```python
from build123d import *

# Parameters (mm, degrees)
SALIENTE_EXTRUIR1_DEPTH = 5
SALIENTE_EXTRUIR2_DEPTH = 10
SALIENTE_EXTRUIR3_DEPTH = 2
CORTAR_EXTRUIR1_START   = 7
CROQUIS2_R              = 2.2
CORTAR_EXTRUIR1_DEPTH   = 14
CROQUIS3_R              = 1.6
CROQUIS3_W              = 5
CROQUIS3_H              = 4
CROQUIS3_W_2            = 2
CORTAR_EXTRUIR2_DEPTH   = 2.4
REDONDEO1_R             = 2
REDONDEO2_R             = 2
REDONDEO3_R             = 1
REDONDEO4_R             = 1.2


with BuildPart() as part:
    # Croquis1 → Saliente-Extruir1 (new body)
    with BuildSketch(Plane(origin=(0, 0, 0), x_dir=(0, 0, -1), z_dir=(1, 0, 0))):
        Polygon((-12.7, 2.4), (-12.7, 0), (12.7, 0), (12.7, 2.4), (7, 2.4), (7, 20), (2, 20), (2, 11.4), (4.4, 11.4), (4.4, 8.6), (2, 8.6), (2, 2.4), (-2, 2.4), (-2, 8.6), (-4.4, 8.6), (-4.4, 11.4), (-2, 11.4), (-2, 20), (-7, 20), (-7, 2.4), align=None)
    extrude(amount=-SALIENTE_EXTRUIR1_DEPTH)

    # Croquis1<3> → Saliente-Extruir2 (add)
    with BuildSketch(Plane(origin=(0, 0, 0), x_dir=(0, 0, -1), z_dir=(1, 0, 0))):
        Polygon((2, 2.4), (7, 2.4), (12.7, 2.4), (12.7, 0), (-12.7, 0), (-12.7, 2.4), (-7, 2.4), (-2, 2.4), align=None)
    extrude(amount=SALIENTE_EXTRUIR2_DEPTH)

    # Croquis1<4> → Saliente-Extruir3 (add)
    with BuildSketch(Plane(origin=(0, 0, 0), x_dir=(0, 0, -1), z_dir=(1, 0, 0))):
        Polygon((-7, 20), (-7, 2.4), (-2, 2.4), (-2, 8.6), (-4.4, 8.6), (-4.4, 11.4), (-2, 11.4), (-2, 20), align=None)
        Polygon((2, 2.4), (7, 2.4), (7, 20), (2, 20), (2, 11.4), (4.4, 11.4), (4.4, 8.6), (2, 8.6), align=None)
    extrude(amount=SALIENTE_EXTRUIR3_DEPTH)

    # Croquis2 → Cortar-Extruir1 (cut)
    with BuildSketch(Plane.XY.offset(CORTAR_EXTRUIR1_START)):
        with Locations(Location((-2, 15, 0), (0, 0, 270))):
            Circle(CROQUIS2_R)
        with Locations(Location((-2, 5, 0), (0, 0, 270))):
            Circle(CROQUIS2_R)
    extrude(amount=-CORTAR_EXTRUIR1_DEPTH, mode=Mode.SUBTRACT)

    # Croquis3 → Cortar-Extruir2 (cut)
    with BuildSketch(Plane(origin=(0, 0, 0), x_dir=(1, 0, 0), z_dir=(0, 1, 0))):
        Polygon((-5, 7), (0, 7), (2, 12.7), (-5, 12.7), align=None)
        Polygon((2, -12.7), (0, -7), (-5, -7), (-5, -12.7), align=None)
        with Locations(Location((6, -8.7, 0), (0, 0, 90))):
            Circle(CROQUIS3_R)
        with Locations(Location((6, 8.7, 0), (0, 0, 90))):
            Circle(CROQUIS3_R)
        with Locations((-2.5, 0)):
            Rectangle(CROQUIS3_W, CROQUIS3_H)
        with Locations((1, 0)):
            Rectangle(CROQUIS3_W_2, CROQUIS3_H)
    extrude(amount=CORTAR_EXTRUIR2_DEPTH, mode=Mode.SUBTRACT)

    # Redondeo1
    redondeo1_edges = [part.edges().sort_by_distance(p)[0] for p in [
        (2, 20, -4.5),
        (2, 20, 4.5),
    ]]
    fillet(redondeo1_edges, radius=REDONDEO1_R)

    # Redondeo2
    # the kernel refuses this fillet: 2 mm, written as the material it adds along each edge
    with BuildSketch(Plane(origin=(2, 2.4, 3), x_dir=(1, 0, 0), z_dir=(0, 0, -1))) as redondeo2_piece_1_section:
        with BuildLine():
            CenterArc((REDONDEO2_R, -REDONDEO2_R), REDONDEO2_R, 90, 90)
            Line((0, -REDONDEO2_R), (0, 0))
            Line((0, 0), (REDONDEO2_R, 0))
        make_face()
    redondeo2_piece_1 = extrude(amount=15, mode=Mode.PRIVATE)
    redondeo2_piece_1 = split(redondeo2_piece_1, bisect_by=Plane(origin=(2, 2.4, 2), z_dir=(0, 0, 1)), keep=Keep.TOP, mode=Mode.PRIVATE)
    add(redondeo2_piece_1)
    with BuildSketch(Plane(origin=(2, 2.4, -2), x_dir=(1, 0, 0), z_dir=(0, 0, -1))) as redondeo2_piece_2:
        with BuildLine():
            CenterArc((REDONDEO2_R, -REDONDEO2_R), REDONDEO2_R, 90, 90)
            Line((0, -REDONDEO2_R), (0, 0))
            Line((0, 0), (REDONDEO2_R, 0))
        make_face()
    extrude(amount=5)
    with BuildSketch(Plane(origin=(-5, 2.4, -7), x_dir=(0, 0, -1), z_dir=(1, 0, 0))) as redondeo2_piece_3_section:
        with BuildLine():
            CenterArc((REDONDEO2_R, REDONDEO2_R), REDONDEO2_R, 180, 90)
            Line((0, REDONDEO2_R), (0, 0))
            Line((0, 0), (REDONDEO2_R, 0))
        make_face()
    redondeo2_piece_3 = extrude(amount=7, mode=Mode.PRIVATE)
    redondeo2_piece_3 = split(redondeo2_piece_3, bisect_by=Plane(origin=(-0.548095369, 2.4, -5.4379282), z_dir=(0.9435999821328808, 0, 0.331087713029081)), keep=Keep.TOP, mode=Mode.PRIVATE)
    redondeo2_piece_3 = redondeo2_piece_3 - Plane(origin=(-2, 5, -7), x_dir=(0, -1, 0), z_dir=(0, 0, 1)) * Cylinder(2.2, 22, mode=Mode.PRIVATE)
    add(redondeo2_piece_3)
    with BuildSketch(Plane(origin=(2, 2.4, 7), x_dir=(0, 1, 0), z_dir=(-1, 0, 0))) as redondeo2_piece_4_section:
        with BuildLine():
            CenterArc((REDONDEO2_R, -REDONDEO2_R), REDONDEO2_R, 90, 90)
            Line((0, -REDONDEO2_R), (0, 0))
            Line((0, 0), (REDONDEO2_R, 0))
        make_face()
    redondeo2_piece_4 = extrude(amount=7, mode=Mode.PRIVATE)
    redondeo2_piece_4 = split(redondeo2_piece_4, bisect_by=Plane(origin=(0.219238147, 2.4, 7.62482872), z_dir=(0.9435999821328808, 0, -0.331087713029081)), keep=Keep.TOP, mode=Mode.PRIVATE)
    redondeo2_piece_4 = redondeo2_piece_4 - Plane(origin=(-2, 5, 7), x_dir=(0, -1, 0), z_dir=(0, 0, 1)) * Cylinder(2.2, 22, mode=Mode.PRIVATE)
    add(redondeo2_piece_4)
    with BuildSketch(Plane(origin=(0, 0, 7), x_dir=(-1, 0, 0), z_dir=(0, 1, 0))) as redondeo2_piece_5:
        with BuildLine():
            CenterArc((REDONDEO2_R * 0.708893916529, REDONDEO2_R), REDONDEO2_R, 199.334808538, 70.665191462)
            Line((-REDONDEO2_R * 0.234706065604, REDONDEO2_R * 0.668912286971), (0, 0))
            Line((0, 0), (REDONDEO2_R * 0.708893916529, 0))
        make_face()
    extrude(amount=2.4)
    with BuildSketch(Plane(origin=(0, 0, -7), x_dir=(-1, 0, 0), z_dir=(0, 1, 0))) as redondeo2_piece_6:
        with BuildLine():
            CenterArc((REDONDEO2_R * 0.708893916529, -REDONDEO2_R), REDONDEO2_R, 90, 70.665191462)
            Line((-REDONDEO2_R * 0.234706065604, -REDONDEO2_R * 0.668912286971), (0, 0))
            Line((0, 0), (REDONDEO2_R * 0.708893916529, 0))
        make_face()
    extrude(amount=2.4)
    with BuildSketch(Plane(origin=(2, 2.4, 7), x_dir=(0, 1, 0), z_dir=(0, 0, -1))) as redondeo2_piece_7:
        with BuildLine():
            CenterArc((REDONDEO2_R, REDONDEO2_R), REDONDEO2_R, 180, 90)
            Line((0, REDONDEO2_R), (0, 0))
            Line((0, 0), (REDONDEO2_R, 0))
        make_face()
    extrude(amount=5)
    with BuildSketch(Plane(origin=(2, 2.4, 12), x_dir=(0, 1, 0), z_dir=(0, 0, -1))) as redondeo2_piece_8_section:
        with BuildLine():
            CenterArc((REDONDEO2_R, REDONDEO2_R), REDONDEO2_R, 180, 90)
            Line((0, REDONDEO2_R), (0, 0))
            Line((0, 0), (REDONDEO2_R, 0))
        make_face()
    redondeo2_piece_8 = extrude(amount=15, mode=Mode.PRIVATE)
    redondeo2_piece_8 = split(redondeo2_piece_8, bisect_by=Plane(origin=(2, 2.4, -2), z_dir=(0, 0, -1)), keep=Keep.TOP, mode=Mode.PRIVATE)
    add(redondeo2_piece_8)
    with BuildSketch(Plane(origin=(2, 2.4, -2), x_dir=(1, 0, 0), z_dir=(0, 0, -1))) as redondeo2_piece_9a_section:
        with BuildLine():
            CenterArc((REDONDEO2_R, -REDONDEO2_R), REDONDEO2_R, 90, 90)
            Line((0, -REDONDEO2_R), (0, 0))
            Line((0, 0), (REDONDEO2_R, 0))
        make_face()
    redondeo2_piece_9a = extrude(amount=10, mode=Mode.PRIVATE)
    redondeo2_piece_9a = split(redondeo2_piece_9a, bisect_by=Plane(origin=(2, 2.4, -7), z_dir=(0, 0, -1)), keep=Keep.TOP, mode=Mode.PRIVATE)
    with BuildSketch(Plane(origin=(-5, 2.4, -7), x_dir=(0, 0, -1), z_dir=(1, 0, 0))) as redondeo2_piece_9b_section:
        with BuildLine():
            CenterArc((REDONDEO2_R, REDONDEO2_R), REDONDEO2_R, 180, 90)
            Line((0, REDONDEO2_R), (0, 0))
            Line((0, 0), (REDONDEO2_R, 0))
        make_face()
    redondeo2_piece_9b = extrude(amount=12, mode=Mode.PRIVATE)
    redondeo2_piece_9b = split(redondeo2_piece_9b, bisect_by=Plane(origin=(2, 2.4, -7), z_dir=(1, 0, 0)), keep=Keep.TOP, mode=Mode.PRIVATE)
    redondeo2_piece_9b = redondeo2_piece_9b - Plane(origin=(6, 2.4, -8.7), x_dir=(0, 0, -1), z_dir=(0, -1, 0)) * Cylinder(1.6, 32, mode=Mode.PRIVATE)
    redondeo2_piece_9 = redondeo2_piece_9a & redondeo2_piece_9b
    add(redondeo2_piece_9)
    with BuildSketch(Plane(origin=(-5, 2.4, -7), x_dir=(0, 0, -1), z_dir=(1, 0, 0))) as redondeo2_piece_10a_section:
        with BuildLine():
            CenterArc((REDONDEO2_R, REDONDEO2_R), REDONDEO2_R, 180, 90)
            Line((0, REDONDEO2_R), (0, 0))
            Line((0, 0), (REDONDEO2_R, 0))
        make_face()
    redondeo2_piece_10a = extrude(amount=7, mode=Mode.PRIVATE)
    redondeo2_piece_10a = split(redondeo2_piece_10a, bisect_by=Plane(origin=(-0.548095369, 2.4, -5.4379282), z_dir=(-0.9435999821328808, 0, -0.331087713029081)), keep=Keep.TOP, mode=Mode.PRIVATE)
    redondeo2_piece_10a = redondeo2_piece_10a - Plane(origin=(-2, 5, -7), x_dir=(0, -1, 0), z_dir=(0, 0, 1)) * Cylinder(2.2, 22, mode=Mode.PRIVATE)
    with BuildSketch(Plane(origin=(0, 0, -7), x_dir=(-1, 0, 0), z_dir=(0, 1, 0))) as redondeo2_piece_10b_section:
        with BuildLine():
            CenterArc((REDONDEO2_R * 0.708893916529, -REDONDEO2_R), REDONDEO2_R, 90, 70.665191462)
            Line((-REDONDEO2_R * 0.234706065604, -REDONDEO2_R * 0.668912286971), (0, 0))
            Line((0, 0), (REDONDEO2_R * 0.708893916529, 0))
        make_face()
    redondeo2_piece_10b = extrude(amount=5.944469583, mode=Mode.PRIVATE)
    redondeo2_piece_10b = split(redondeo2_piece_10b, bisect_by=Plane(origin=(0, 2.4, -7), z_dir=(0, 1, 0)), keep=Keep.TOP, mode=Mode.PRIVATE)
    redondeo2_piece_10b = redondeo2_piece_10b - Plane(origin=(-2, 5, -7), x_dir=(0, -1, 0), z_dir=(0, 0, 1)) * Cylinder(2.2, 18, mode=Mode.PRIVATE)
    redondeo2_piece_10 = redondeo2_piece_10a & redondeo2_piece_10b
    add(redondeo2_piece_10)
    with BuildSketch(Plane(origin=(7, 2.4, 7), x_dir=(0, 1, 0), z_dir=(-1, 0, 0))) as redondeo2_piece_11a_section:
        with BuildLine():
            CenterArc((REDONDEO2_R, -REDONDEO2_R), REDONDEO2_R, 90, 90)
            Line((0, -REDONDEO2_R), (0, 0))
            Line((0, 0), (REDONDEO2_R, 0))
        make_face()
    redondeo2_piece_11a = extrude(amount=12, mode=Mode.PRIVATE)
    redondeo2_piece_11a = split(redondeo2_piece_11a, bisect_by=Plane(origin=(2, 2.4, 7), z_dir=(1, 0, 0)), keep=Keep.TOP, mode=Mode.PRIVATE)
    redondeo2_piece_11a = redondeo2_piece_11a - Plane(origin=(6, 2.4, 8.7), x_dir=(0, 0, -1), z_dir=(0, -1, 0)) * Cylinder(1.6, 32, mode=Mode.PRIVATE)
    with BuildSketch(Plane(origin=(2, 2.4, 12), x_dir=(0, 1, 0), z_dir=(0, 0, -1))) as redondeo2_piece_11b_section:
        with BuildLine():
            CenterArc((REDONDEO2_R, REDONDEO2_R), REDONDEO2_R, 180, 90)
            Line((0, REDONDEO2_R), (0, 0))
            Line((0, 0), (REDONDEO2_R, 0))
        make_face()
    redondeo2_piece_11b = extrude(amount=10, mode=Mode.PRIVATE)
    redondeo2_piece_11b = split(redondeo2_piece_11b, bisect_by=Plane(origin=(2, 2.4, 7), z_dir=(0, 0, 1)), keep=Keep.TOP, mode=Mode.PRIVATE)
    redondeo2_piece_11 = redondeo2_piece_11a & redondeo2_piece_11b
    add(redondeo2_piece_11)
    with BuildSketch(Plane(origin=(2, 2.4, 7), x_dir=(0, 1, 0), z_dir=(-1, 0, 0))) as redondeo2_piece_12a_section:
        with BuildLine():
            CenterArc((REDONDEO2_R, -REDONDEO2_R), REDONDEO2_R, 90, 90)
            Line((0, -REDONDEO2_R), (0, 0))
            Line((0, 0), (REDONDEO2_R, 0))
        make_face()
    redondeo2_piece_12a = extrude(amount=7, mode=Mode.PRIVATE)
    redondeo2_piece_12a = split(redondeo2_piece_12a, bisect_by=Plane(origin=(0.219238147, 2.4, 7.62482872), z_dir=(-0.9435999821328808, 0, 0.331087713029081)), keep=Keep.TOP, mode=Mode.PRIVATE)
    redondeo2_piece_12a = redondeo2_piece_12a - Plane(origin=(-2, 5, 7), x_dir=(0, -1, 0), z_dir=(0, 0, 1)) * Cylinder(2.2, 22, mode=Mode.PRIVATE)
    with BuildSketch(Plane(origin=(0, 0, 7), x_dir=(-1, 0, 0), z_dir=(0, 1, 0))) as redondeo2_piece_12b_section:
        with BuildLine():
            CenterArc((REDONDEO2_R * 0.708893916529, REDONDEO2_R), REDONDEO2_R, 199.334808538, 70.665191462)
            Line((-REDONDEO2_R * 0.234706065604, REDONDEO2_R * 0.668912286971), (0, 0))
            Line((0, 0), (REDONDEO2_R * 0.708893916529, 0))
        make_face()
    redondeo2_piece_12b = extrude(amount=5.944469583, mode=Mode.PRIVATE)
    redondeo2_piece_12b = split(redondeo2_piece_12b, bisect_by=Plane(origin=(0, 2.4, 7), z_dir=(0, 1, 0)), keep=Keep.TOP, mode=Mode.PRIVATE)
    redondeo2_piece_12b = redondeo2_piece_12b - Plane(origin=(-2, 5, 7), x_dir=(0, -1, 0), z_dir=(0, 0, 1)) * Cylinder(2.2, 18, mode=Mode.PRIVATE)
    redondeo2_piece_12 = redondeo2_piece_12a & redondeo2_piece_12b
    add(redondeo2_piece_12)

    # Redondeo3
    redondeo3_edges = [part.edges().sort_by_distance(p)[0] for p in [
        (2, 1.2, 2),
        (2, 1.2, -2),
    ]]
    fillet(redondeo3_edges, radius=REDONDEO3_R)

    # Redondeo4
    redondeo4_edges = [part.edges().sort_by_distance(p)[0] for p in [
        (-1.5, 11.4, 4.4),
        (-1.5, 8.6, 4.4),
        (-1.5, 8.6, -4.4),
        (-1.5, 11.4, -4.4),
    ]]
    fillet(redondeo4_edges, radius=REDONDEO4_R)


solid = part.part
```
Geometry check sheet. Reference: the model listing, model coordinates, mm. A direction names the side the tool comes from. Round coordinates to 2 decimals unless told otherwise and drop trailing zeros. Order: outer loops, then holes, each group sorted by start corner. A loop starts at its lowest first (then second) coordinate and runs counter-clockwise, first axis right, second up. Notation, with made-up numbers: (-2.5, 66.25) -> (12.5, 66.25) arc R23 cw to (12.5, 101.25) -> close; hole circle Ø4 at (83.25, 48). An arc over 180 degrees is marked (long way). Return JSON: item names as keys, results as strings. Group by question number.
Q1. Release check for a two-part mould opening along Z. For faces 1 (the flat face through (1.224, 1.239, 10.488)), 2 (the cylindrical face through (-1.451, 8.961, -4.058)), 3 (the flat face through (-1, 10, -7)), 4 (the cylindrical face through (2.6, 2.97, -4.67)) record: released by +Z, released by -Z, zero draft, split by the parting line, or undercut.
Q2. Section check D-D, the plane x = -2. Count the separate pieces of the cut face and the enclosed holes in it, plus the area to 3 significant figures.
Q3. Material ranges on probe 1 along Z at (x, y) = (6, 1.7); probe 2 along X at (y, z) = (5, 5.9); probe 3 along Y at (x, z) = (-0.75, -4.25), recorded low to high. Write a range as from..to.
Q4. Section check B-B, the plane x = 6. Record the boundary of the cut face in (y, z).
Q5. Section check A-A, the plane y = 15. Record the boundary of the cut face in (x, z), plus the area to 3 significant figures.
Q6. Gauge pin test, flat ends, axial feed: pin 1 (4 mm diameter, centred on y = 12.5, z = -3.5, fed in from +X); pin 2 (4.5 mm diameter, centred on x = 1, y = 5.5, fed in from -Z); pin 3 (5.5 mm diameter, centred on x = -2, y = 5, fed in from -Z); pin 4 (1 mm diameter, centred on x = 7.5, y = 4.5, fed in from -Z) (3 decimals). Record the tip position at first contact, or that the pin passes through.
Q7. Section check C-C, the plane z = -4. Record the boundary of the cut face in (x, y).
Q8. Tool access check on faces 5 (the flat face through (2, 11.3, 4.5)), 6 (the flat face through (0, 17, -2)), 7 (the flat face through (-2, 11.4, 3)). Record the directions out of +Z, -Z, +X, -X, +Y, -Y that give a thin tool (end or side, any length) a straight path to the whole face; none if there is none.
Numbers:
{
 "1": {"face 1": "released by +Z", "face 2": "undercut", "face 3": "released by -Z", "face 4": "zero draft"},
 "2": {"separate pieces": "6", "enclosed holes": "0", "area": "99.8 mm^2"},
 "3": {"probe 1": "-12.7..-10.3, -7.1..7.1, 10.3..12.7", "probe 2": "-5..-4.2, 0.2..2", "probe 3": "0..3.19, 6.81..9.22, 10.78..13.19, 16.81..20"},
 "4": {"outline": "(0, -12.7) -> (2.4, -12.7) -> (2.4, -10.3) -> (0, -10.3) -> close; (0, -7.1) -> (2.4, -7.1) -> (2.4, 7.1) -> (0, 7.1) -> close; (0, 10.3) -> (2.4, 10.3) -> (2.4, 12.7) -> (0, 12.7) -> close"},
 "5": {"outline": "(-5, -7) -> (-4.2, -7) -> (-4.2, -2) -> (-5, -2) -> close; (-5, 2) -> (-4.2, 2) -> (-4.2, 7) -> (-5, 7) -> close; (0.2, -7) -> (2, -7) -> (2, -2) -> (0.2, -2) -> close; (0.2, 2) -> (2, 2) -> (2, 7) -> (0.2, 7) -> close", "area": "26.0 mm^2"},
 "6": {"pin 1": "x = 2", "pin 2": "z = -7.36", "pin 3": "z = -7.53", "pin 4": "through"},
 "7": {"outline": "(-5, 0) -> (10, 0) -> (10, 2.4) -> (4, 2.4) arc R2 cw to (2, 4.4) -> (2, 8.91) -> (-5, 8.91) -> close; (-5, 11.09) -> (2, 11.09) -> (2, 18) arc R2 ccw to (0, 20) -> (-5, 20) -> close; hole circle Ø4.4 at (-2, 5); hole circle Ø4.4 at (-2, 15)"},
 "8": {"face 5": "+Z, -Z, +X, +Y", "face 6": "+X, -X, +Y", "face 7": "+X, -X"}
}
